Could you check a few things on this drawing? It's one solid part, dimensions in mm from its lowest x, y, z. A direction names the side the tool comes from. Round coordinates to 2 decimals unless told otherwise and drop trailing zeros. Order: outer loops, then holes, each group sorted by start corner. A loop starts at its lowest first (then second) coordinate and runs counter-clockwise, first axis right, second up. Notation, with made-up numbers: M -32.5,-36 L -0.5,-36 A8 ccw -0.5,-25 Z; hole C 68.5,20 d2. An arc over 180 degrees is marked long. Answer as CSV lines item,"result". Start each with the question number.
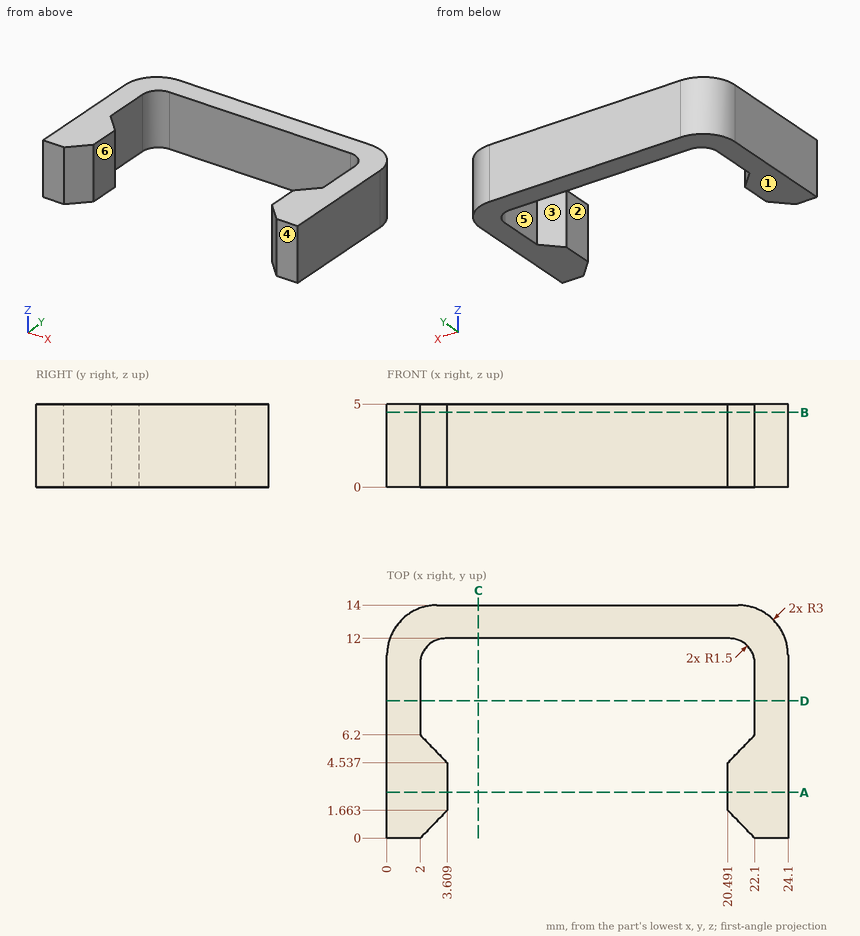
Item 1: If we section it at D-D on y = 8.25: Please give me the cut outline in (x, z).
Item 2: For P1, Ø1, axis at x = 20.5, z = 1.5, coming from the -Y side, with a flat end and sliding along its axis, tell me the tip position at first contact or that it passes through.
Item 3: We'd pull the mould along Y, two halves only. Please class the marked faces 4, 5 and 6: pulls with the +Y half, pulls with the -Y half, needs draft (parallel to the pull), parting line crosses it, or undercut.
Item 4: If I drill on line 1 along X through (y, z) = (2, 3.55); line 2 along X through (y, z) = (9.5, 4.6); line 3 along Y through (x, z) = (17.5, 1.8), over which ranges is the centre line in solid material (lowest first)?
Item 5: If we section it at B-B on z = 4.5: Please give me the cut outline in (x, y), and give its area (3 significant figures).
Item 6: Which directions (+Z, -Z, +X, -X, +Y, -Y) give clear straight access to the entire face, cutting with the end or side of a thin tool? Please do the marked faces 1, 2 and 3.
Item 7: If we section it at C-C on x = 5.5: Please give me the cut outline in (y, z), and give its area (3 significant figures).
Item 8: If we section it at A-A on y = 2.75: Please give me the cut outline in (x, z).
Geometry says:
1,outline,"M 0,0 L 2,0 L 2,5 L 0,5 Z; M 22.1,0 L 24.1,0 L 24.1,5 L 22.1,5 Z"
2,P1,"y = 1.14"
3,face 4,"pulls with the -Y half"
3,face 5,"undercut"
3,face 6,"needs draft"
4,line 1,"0 to 3.61, 20.49 to 24.1"
4,line 2,"0 to 2, 22.1 to 24.1"
4,line 3,"12 to 14"
5,outline,"M 0,0 L 2,0 L 3.61,1.66 L 3.61,4.54 L 2,6.2 L 2,10.5 A1.5 cw 3.5,12 L 20.6,12 A1.5 cw 22.1,10.5 L 22.1,6.2 L 20.49,4.54 L 20.49,1.66 L 22.1,0 L 24.1,0 L 24.1,11 A3 ccw 21.1,14 L 3,14 A3 ccw 0,11 Z"
5,area,"108 mm²"
6,face 1,"-Z, +X, -X, +Y, -Y"
6,face 2,"+Z, -Z, -Y"
6,face 3,"+Z, -Z"
7,outline,"M 12,0 L 14,0 L 14,5 L 12,5 Z"
7,area,"10.0 mm²"
8,outline,"M 0,0 L 3.61,0 L 3.61,5 L 0,5 Z; M 20.49,0 L 24.1,0 L 24.1,5 L 20.49,5 Z"
